Autodesk Inventor part; units mm, degrees
ref_plane "YZ Plane" through (0, 0, 0) normal (1, 0, 0) x (0, 1, 0)
ref_plane "XZ Plane" through (0, 0, 0) normal (0, 1, 0) x (-1, 0, 0)
ref_plane "XY Plane" through (0, 0, 0) normal (0, 0, 1) x (1, 0, 0)
sketch "Sketch1" plane through (0, 0, 0) normal (0, 1, 0) x (-1, 0, 0)
  line L0 (72.5, -45) -> (-72.5, -45)
  line L1 (-72.5, -45) -> (-72.5, 45)
  line L2 (-72.5, 45) -> (72.5, 45)
  line L3 (72.5, 45) -> (72.5, -45)
  line L4 (72.5, -45) -> (-72.5, 45) construction
  line L5 (-72.5, -45) -> (72.5, 45) construction
  point P0 (0, 0)
  dimension "d0" = 145
  dimension "d1" = 90
extrude "Extrusion1" add sketch "Sketch1" along normal blind 3
sketch "Sketch4" plane through (72.5, 0, -45) normal (0, 0, -1) x (-1, 0, 0)
  line L0 (35, 3) -> (110, 3)
  line L1 (110, 3) -> (110, 0)
  line L2 (110, 0) -> (35, 0)
  line L3 (35, 0) -> (35, 3)
  line L4 (35, 3) -> (110, 0) construction
  line L5 (110, 3) -> (35, 0) construction
  line L6 (0, 3) -> (145, 3)
  point P0 (72.5, 0)
  point P1 (72.5, 1.5)
  dimension "d28" = 75
  dimension "d29" = 3
  dimension "d30" = 0
extrude "Extrusion3" add sketch "Sketch4" along normal blind 50
sketch "Sketch3" plane through (0, 3, 0) normal (0, 1, 0) x (1, 0, 0)
  circle A0 centre (62.5, -34.9998) radius 2.5
  circle A1 centre (-62.5, -35) radius 2.5
  circle A2 centre (-39.5, 24.592) radius 2.5
  circle A3 centre (39.5, 24.5944) radius 2.5
  line L0 (-72.5, 45) -> (-72.5, -45)
  line L1 (-72.5, -45) -> (72.5, -45)
  point P0 (0, 0)
  dimension "d4" = 5
  dimension "d7" = 5
  dimension "d10" = 5
  dimension "d13" = 5
  dimension "d20" = 79
  dimension "d21" = 125
  dimension "d22" = 23
  dimension "d23" = 59.592
  dimension "d24" = 10
  dimension "d25" = 10
extrude "Extrusion2" cut sketch "Sketch3" against normal through all
fillet "Fillet1" radius 6 4 edges at (72.5, 1.5, 45) (-72.5, 1.5, 45) (-37.5, 1.5, -95) (37.5, 1.5, -95)
fillet "Fillet2" radius 17.5 4 edges at (72.5, 1.5, -45) (-72.5, 1.5, -45) (37.5, 1.5, -45) (-37.5, 1.5, -45)
properties part number "chasis_arriba"
Work out the finished part from the listing and answer in its coordinate system (mm). Coordinates: 2 decimals unless noted, no trailing zeros. Order: outer loops, then holes, each group sorted by start corner. A loop starts at its lowest first (then second) coordinate and runs counter-clockwise, first axis right, second up. Notation, with made-up numbers: (30.5, -37.75) - (42.5, -37.75) arc R27 cw to (42.5, -4.75) - close; hole circle Ø10 at (76, -35). An arc over 180 degrees is marked (long way). Answer as a JSON object with one key per item and string values.
1. The mould has two halves that part along Z. Classify faces 1 (the face through (-60.115, 1.521, 34.249)), 2 (the face through (1, 0, -8)), 3 (the face through (67.51, 1.52, -39.74)), 4 (the face through (-38.156, 1.521, -26.7)): +Z half, -Z half, draft (parallel to the pull), parting line (faces both ways), or undercut.
Output values:
{"face 1": "undercut", "face 2": "draft", "face 3": "-Z half", "face 4": "undercut"}
2. Each of these flat-tipped pins is pushed along its axis until it touches: P1, Ø8, axis at x = -39.5, z = -24.592, coming from the -Y side; P2, Ø1.5, axis at y = 2, z = -66.5, coming from the -X side. Where does it stop, or does it pass through?
Output values:
{"P1": "stops at y = 0", "P2": "stops at x = -37.5"}
3. Find section B-B on y = 1.5. Count the separate pieces of the cut face and the enclosed holes in it, plus the area to 3 significant figures.
Output values:
{"separate pieces": "1", "enclosed holes": "4", "area": "16,700 mm²"}
4. Find section D-D on z = -52. Determine the outline of the cut face in (x, y), plus the area to 3 significant figures.
Output values:
{"outline": "(-41, 0) - (41, 0) - (41, 3) - (-41, 3) - close", "area": "246 mm²"}
5. Find section A-A on x = -62.5. Determine the outline of the cut face in (y, z).
Output values:
{"outline": "(0, -43.31) - (3, -43.31) - (3, 32.5) - (0, 32.5) - close; (0, 37.5) - (3, 37.5) - (3, 45) - (0, 45) - close"}
6. Find section C-C on x = -39.5. Determine the outline of the cut face in (y, z), plus the area to 3 significant figures.
Output values:
{"outline": "(0, -54.38) - (3, -54.38) - (3, -27.09) - (0, -27.09) - close; (0, -22.09) - (3, -22.09) - (3, 45) - (0, 45) - close", "area": "283 mm²"}
7. Consider line 1 (X direction, y = 1.8, z = 35); line 2 (X direction, y = 0.8, z = -25); line 3 (X direction, y = 1.95, z = -74). Determine where each line is inside the solid, lowest interval first.
Output values:
{"line 1": "x = -72.5 to -65, -60 to 60, 65 to 72.5", "line 2": "x = -72.5 to -41.97, -37.03 to 37.03, 41.97 to 72.5", "line 3": "x = -37.5 to 37.5"}
